```python
from build123d import *

# Parameters (mm, degrees)
SKETCH_1_R          = 4
SKETCH_1_R_2        = 1.55
SKETCH_1_W          = 28
SKETCH_1_H          = 8
EXTRUDE_1_DEPTH     = 2
SKETCH_2_R          = 4
CUT_EXTRUDE_1_DEPTH = 10
FILLET_2_R          = 1


with BuildPart() as part:
    # 草图1 → 凸台-拉伸1 (new body)
    with BuildSketch(Plane.XY):
        Polygon((-80, 0), (0, 0), (13.5, 6.295153385), (13.5, 30), (33.5, 30), (33.5, 45), (3.5, 45), (0, 48.5), (-25, 48.5), (-34.361702128, 44.5), (-35.671585242, 43.940322669), (-80, 25), align=None)
        with Locations((-66, 6.5)):
            Circle(SKETCH_1_R, mode=Mode.SUBTRACT)
        with Locations((-46, 6.5)):
            Circle(SKETCH_1_R, mode=Mode.SUBTRACT)
        with Locations((-76, 12.5)):
            Circle(SKETCH_1_R_2, mode=Mode.SUBTRACT)
        with Locations((-56, 12.5)):
            Circle(SKETCH_1_R_2, mode=Mode.SUBTRACT)
        with Locations((-36, 12.5)):
            Circle(SKETCH_1_R_2, mode=Mode.SUBTRACT)
        with Locations((-26, 6.5)):
            Circle(SKETCH_1_R, mode=Mode.SUBTRACT)
        with Locations((-6, 6.5)):
            Circle(SKETCH_1_R, mode=Mode.SUBTRACT)
        with Locations((-16, 12.5)):
            Circle(SKETCH_1_R_2, mode=Mode.SUBTRACT)
        with Locations((-42, 33)):
            Circle(SKETCH_1_R_2, mode=Mode.SUBTRACT)
        with Locations((-32.5, 32.5)):
            Circle(SKETCH_1_R_2, mode=Mode.SUBTRACT)
        with Locations((-12.5, 25)):
            Rectangle(SKETCH_1_W, SKETCH_1_H, mode=Mode.SUBTRACT)
        with Locations((-20, 33)):
            Circle(SKETCH_1_R_2, mode=Mode.SUBTRACT)
        with Locations((-5, 33)):
            Circle(SKETCH_1_R_2, mode=Mode.SUBTRACT)
        with Locations((7.5, 32.5)):
            Circle(SKETCH_1_R_2, mode=Mode.SUBTRACT)
        with Locations((29.5, 33.5)):
            Circle(SKETCH_1_R_2, mode=Mode.SUBTRACT)
        with Locations((-20, 45)):
            Circle(SKETCH_1_R_2, mode=Mode.SUBTRACT)
        with Locations((-5, 45)):
            Circle(SKETCH_1_R_2, mode=Mode.SUBTRACT)
        with BuildLine():
            ThreePointArc((13.5, 33.791900756), (11.07365329, 38.26406905), (15, 41.5))
            Line((15, 41.5), (20.5, 41.5))
            ThreePointArc((20.5, 41.5), (24.5, 37.5), (20.5, 33.5))
            Line((20.5, 33.5), (15, 33.5))
            ThreePointArc((15, 33.5), (14.23593095, 33.57365329), (13.5, 33.791900756))
        make_face(mode=Mode.SUBTRACT)
        with Locations((29.5, 41.5)):
            Circle(SKETCH_1_R_2, mode=Mode.SUBTRACT)
    extrude(amount=EXTRUDE_1_DEPTH)

    # 草图2 → 切除-拉伸1 (cut)
    with BuildSketch(Plane.XY.offset(2)):
        with Locations((3.464101615, 50.5)):
            Circle(SKETCH_2_R)
        with Locations((-28.464101615, 50.5)):
            Circle(SKETCH_2_R)
    extrude(amount=-CUT_EXTRUDE_1_DEPTH, mode=Mode.SUBTRACT)

    # 圆角2
    fillet_2_edges = [part.edges().sort_by_distance(p)[0] for p in [
        (1.464101615, 47.035898385, 1),
        (-29.413394303, 46.614276979, 1),
        (1.5, 21, 1),
        (1.5, 29, 1),
        (-26.5, 29, 1),
        (-26.5, 21, 1),
        (13.5, 6.295153385, 1),
        (0, 0, 1),
        (-80, 0, 1),
        (-80, 25, 1),
        (-25, 48.5, 1),
        (0, 48.5, 1),
    ]]
    fillet(fillet_2_edges, radius=FILLET_2_R)


solid = part.part
```
CAD build for the part. Positions are in the model's coordinates, mm. A direction names the side the tool comes from. Give positions to 0.01 mm unless a question says otherwise; leave off trailing zeros. Write each loop counter-clockwise with the first axis right and the second up, starting at its lowest first coordinate (ties: lowest second). Pieces come first, ordered by that corner, then holes. Notation, with made-up numbers: M 80,6 L 92,6 A30 cw 92,35 Z; hole C 73.25,41.5 d8. An arc over 180 degrees is marked long. Return JSON: item names as keys, results as strings. Group by question number.
(1) Band-saw the part on C-C (y = 37). Give the cut face in (x, z), and give its area (3 significant figures).
(2) Band-saw the part on A-A (x = 29.5). Give the cut face in (y, z), and give its area (3 significant figures).
(3) Flat gauge pins, fed straight in: pin 1 Ø8 at (x, y) = (-1, 12) entering from -Z; pin 2 Ø1.9 at (x, y) = (-20, 33) entering from +Z; pin 3 Ø1 at (x, z) = (18.5, 1) entering from +Y. Where does each tip first touch, or does it go through?
(4) 3-axis set-ups, long thin cutter, end or side, ignore diameter. For faces 5 (the face through (-26.5, 25, 1)), 6 (the face through (-37, 25, 2)): which of +Z, -Z, +X, -X, +Y, -Y reach the whole face in a straight line?
(5) Mould opens along Y. For faces 1 (the face through (19, 45, 1)), 2 (the face through (-80, 13, 1)), 3 (the face through (-17.55, 12.57, 0.99)), 4 (the face through (-13, 21, 1)) say: pulls with the +Y half, pulls with the -Y half, needs draft (parallel to the pull), parting line crosses it, or undercut.
(6) Band-saw the part on B-B (x = -46). Give the cut face in (y, z).
(7) Band-saw the part on D-D (z = 0.55). State how many separate pieces and enclosed holes the cut face has, and give its area (3 significant figures).
(8) Drill centre lines: L1, parallel to Y at x = -1, z = 1.45; L2, parallel to X at y = 13.5, z = 1.55; L3, parallel to X at y = 5, z = 1.3. Where is each one in solid material? Low to high. Write a range as [from, to].
Entries:
{
 "1": {"outline": "M -51.91,0 L 11.03,0 L 11.03,2 L -51.91,2 Z; M 24.47,0 L 33.5,0 L 33.5,2 L 24.47,2 Z", "area": "144 mm^2"},
 "2": {"outline": "M 30,0 L 31.95,0 L 31.95,2 L 30,2 Z; M 35.05,0 L 39.95,0 L 39.95,2 L 35.05,2 Z; M 43.05,0 L 45,0 L 45,2 L 43.05,2 Z", "area": "17.6 mm^2"},
 "3": {"pin 1": "stops at z = 0", "pin 2": "passes through", "pin 3": "stops at y = 45"},
 "4": {"face 5": "+Z, -Z", "face 6": "+Z, +X, -X, +Y, -Y"},
 "5": {"face 1": "pulls with the +Y half", "face 2": "needs draft", "face 3": "undercut", "face 4": "undercut"},
 "6": {"outline": "M 0,0 L 2.5,0 L 2.5,2 L 0,2 Z; M 10.5,0 L 39.53,0 L 39.53,2 L 10.5,2 Z"},
 "7": {"separate pieces": "1", "enclosed holes": "19", "area": "3,490 mm^2"},
 "8": {"L1": "y = [0, 21], [29, 48.5]", "L2": "x = [-80, -77.18], [-74.82, -57.18], [-54.82, -37.18], [-34.82, -17.18], [-14.82, 13.5]", "L3": "x = [-80, -69.71], [-62.29, -49.71], [-42.29, -29.71], [-22.29, -9.71], [-2.29, 10.72]"}
}
